Read the model definition and answer for the solid it produces. Units are mm, in the model's axes. Coordinates: 2 decimals unless noted, no trailing zeros. Write each loop counter-clockwise with the first axis right and the second up, starting at its lowest first coordinate (ties: lowest second). Pieces come first, ordered by that corner, then holes.
Item 1: Section C-C (z = -60) is taken. Give the vertices of the cut face in (x, y) (3 decimals), then the cut area to 3 significant figures.
Item 2: Section B-B (x = -34) is taken. Give the vertices of the cut face in (y, z) (3 decimals), then the cut area to 3 significant figures.
Item 3: Each of these flat-tipped pins is pushed along its axis until it touches: P1, Ø10, axis at x = 5.65, z = -53.34, coming from the +Y side (3 decimals); P2, Ø1, axis at y = 7.5, z = 74, coming from the -X side; P3, Ø5, axis at x = -40.5, y = 4, coming from the +Z side; P4, Ø5, axis at x = 38.5, y = 1.5, coming from the -Z side. Where does it stop, or does it pass through?
Item 4: Section A-A (z = 0) is taken. Give the vertices of the cut face in (x, y) (3 decimals).
Item 5: Section D-D (y = 7.5) is taken. State how many separate pieces and enclosed holes the cut face has, then the cut area to 3 significant figures.
Item 6: Straight lines are drawn through the part: probe 1 along Z at (x, y) = (57, 6); probe 2 along X at (y, z) = (1, 87); probe 3 along X at (y, z) = (7.75, 84.5). For each, find the intervals that lie inside material, in ascending order.
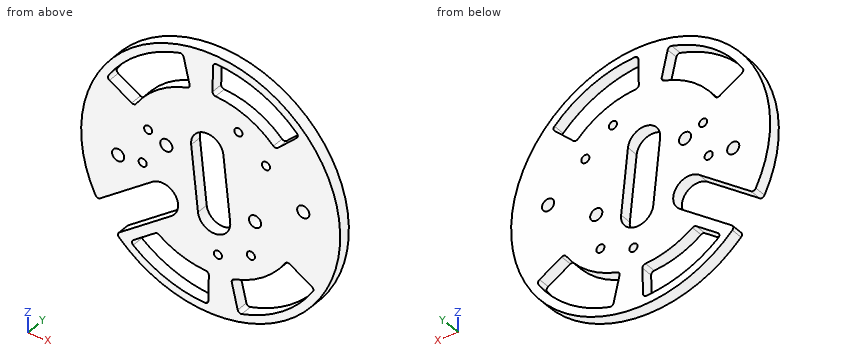
from build123d import *

# Parameters (mm, degrees)
SKETCH1_R           = 101.6
BOSS_EXTRUDE1_DEPTH = 9.525
SKETCH2_R           = 4.7625
SKETCH2_R_2         = 3.175
CUT_EXTRUDE1_DEPTH  = 22.86
SKETCH3_R           = 4.7625
CUT_EXTRUDE2_DEPTH  = 10.525
FILLET1_R           = 2.54
FILLET3_R           = 2.54


with BuildPart() as part:
    # Sketch1 → Boss-Extrude1 (new body)
    with BuildSketch(Plane(origin=(0, 0, 0), x_dir=(1, 0, 0), z_dir=(0, 1, 0))):
        Circle(SKETCH1_R)
    extrude(amount=BOSS_EXTRUDE1_DEPTH)

    # Sketch2 → Cut-Extrude1 (cut)
    with BuildSketch(Plane(origin=(0, 9.525, 0), x_dir=(1, 0, 0), z_dir=(0, 1, 0))):
        with BuildLine():
            Line((-9.955759688, 26.595729902), (-15.303128109, -23.922045692))
            ThreePointArc((-15.303128109, -23.922045692), (-4.010526316, -37.888331696), (9.955759688, -26.595729902))
            Line((9.955759688, -26.595729902), (15.303128109, 23.922045692))
            ThreePointArc((15.303128109, 23.922045692), (4.010526316, 37.888331696), (-9.955759688, 26.595729902))
        make_face()
        with Locations((34.817520913, 15.470948176)):
            Circle(SKETCH2_R)
        with Locations((-34.817520913, -15.470948176)):
            Circle(SKETCH2_R)
        with BuildLine():
            Line((-30.765292524, 38.093536125), (-87.237043764, 79.186441231))
            Line((-87.237043764, 79.186441231), (-104.485964967, 60.325))
            Line((-104.485964967, 60.325), (-45.710214871, 17.555539727))
            ThreePointArc((-45.710214871, 17.555539727), (-27.968755498, 20.352076753), (-30.765292524, 38.093536125))
        make_face()
        with Locations((5.646300897, 53.341856998)):
            Circle(SKETCH2_R_2)
        with Locations((31.560768513, 43.372252797)):
            Circle(SKETCH2_R_2)
        with Locations((-53.341856998, 5.646300897)):
            Circle(SKETCH2_R_2)
        with Locations((43.372252797, -31.560768513)):
            Circle(SKETCH2_R_2)
        with Locations((-49.018553694, -21.781088485)):
            Circle(SKETCH2_R_2)
        with Locations((21.781088485, -49.018553694)):
            Circle(SKETCH2_R_2)
    extrude(amount=-CUT_EXTRUDE1_DEPTH, mode=Mode.SUBTRACT)

    # Sketch3 → Cut-Extrude2 (cut, through all)
    with BuildSketch(Plane(origin=(0, 9.525, 0), x_dir=(1, 0, 0), z_dir=(0, 1, 0))):
        with BuildLine():
            ThreePointArc((15.979287148, 67.997682918), (41.099184753, 56.47901834), (59.78603337, 36.119976659))
            Line((59.78603337, 36.119976659), (81.526409141, 49.254513627))
            ThreePointArc((81.526409141, 49.254513627), (56.044342845, 77.016843191), (21.78993702, 92.72411307))
            Line((21.78993702, 92.72411307), (15.979287148, 67.997682918))
        make_face()
        with BuildLine():
            ThreePointArc((50.898077232, -47.837310063), (28.362672287, -63.832447241), (1.387800686, -69.83621202))
            Line((1.387800686, -69.83621202), (1.892455481, -95.231198209))
            ThreePointArc((1.892455481, -95.231198209), (38.6763713, -87.044246238), (69.406468953, -65.232695541))
            Line((69.406468953, -65.232695541), (50.898077232, -47.837310063))
        make_face()
        with BuildLine():
            ThreePointArc((-15.979287148, -67.997682918), (-41.099184753, -56.47901834), (-59.78603337, -36.119976659))
            Line((-59.78603337, -36.119976659), (-81.526409141, -49.254513627))
            ThreePointArc((-81.526409141, -49.254513627), (-56.044342845, -77.016843191), (-21.78993702, -92.72411307))
            Line((-21.78993702, -92.72411307), (-15.979287148, -67.997682918))
        make_face()
        with BuildLine():
            ThreePointArc((-42.080853774, 55.751450615), (-22.846796408, 66.00792675), (-1.387800686, 69.83621202))
            Line((-1.387800686, 69.83621202), (-1.892455481, 95.231198209))
            ThreePointArc((-1.892455481, 95.231198209), (-34.737758173, 88.689631058), (-63.288565419, 71.183705911))
            Line((-63.288565419, 71.183705911), (-42.080853774, 55.751450615))
        make_face()
        with Locations((-72.619302416, 7.686842105)):
            Circle(SKETCH3_R)
        with Locations((72.619302416, -7.686842105)):
            Circle(SKETCH3_R)
    extrude(amount=-CUT_EXTRUDE2_DEPTH, mode=Mode.SUBTRACT)

    # Fillet1
    fillet1_edges = [part.edges().sort_by_distance(p)[0] for p in [
        (-74.035185173, 4.7625, -69.579820037),
        (-88.980107519, 4.7625, -49.041823639),
    ]]
    fillet(fillet1_edges, radius=FILLET1_R)

    # Fillet3
    fillet3_edges = [part.edges().sort_by_distance(p)[0] for p in [
        (-15.979287148, 4.7625, 67.997682918),
        (-21.78993702, 4.7625, 92.72411307),
        (-81.526409141, 4.7625, 49.254513627),
        (-59.78603337, 4.7625, 36.119976659),
        (50.898077232, 4.7625, 47.837310063),
        (69.406468953, 4.7625, 65.232695541),
        (1.892455481, 4.7625, 95.231198209),
        (1.387800686, 4.7625, 69.83621202),
        (15.979287148, 4.7625, -67.997682918),
        (21.78993702, 4.7625, -92.72411307),
        (81.526409141, 4.7625, -49.254513627),
        (59.78603337, 4.7625, -36.119976659),
        (-42.080853774, 4.7625, -55.751450615),
        (-63.288565419, 4.7625, -71.183705911),
        (-1.892455481, 4.7625, -95.231198209),
        (-1.387800686, 4.7625, -69.83621202),
    ]]
    fillet(fillet3_edges, radius=FILLET3_R)


solid = part.part
Established:
1. outline: (-60.87, 0) - (-47.919, 0) - (-47.919, 9.525) - (-60.87, 9.525) - close; (-35.763, 0) - (35.763, 0) - (35.763, 9.525) - (-35.763, 9.525) - close; (73.977, 0) - (81.991, 0) - (81.991, 9.525) - (73.977, 9.525) - close
1. area: 881 mm2
2. outline: (0, -95.742) - (9.525, -95.742) - (9.525, -88.975) - (0, -88.975) - close; (0, -61.017) - (9.525, -61.017) - (9.525, -40.447) - (0, -40.447) - close; (0, -15.852) - (9.525, -15.852) - (9.525, 10.779) - (0, 10.779) - close; (0, 20.163) - (9.525, 20.163) - (9.525, 61.017) - (0, 61.017) - close; (0, 88.975) - (9.525, 88.975) - (9.525, 95.742) - (0, 95.742) - close
2. area: 968 mm2
3. P1: stops at y = 9.525
3. P2: stops at x = -70.14
3. P3: stops at z = 94.23
3. P4: stops at z = -95.01
4. outline: (-101.6, 0) - (-12.771, 0) - (-12.771, 9.525) - (-101.6, 9.525) - close; (12.771, 0) - (101.6, 0) - (101.6, 9.525) - (12.771, 9.525) - close
5. separate pieces: 1
5. enclosed holes: 15
5. area: 22,100 mm2
6. probe 1: z = -84.1 to -76.31, -40.37 to 53.57, 76.31 to 84.1
6. probe 2: x = -52.47 to -38.78, -20.44 to 1.73, 38.78 to 52.47
6. probe 3: x = -56.41 to -43.96, -19.86 to 1.68, 43.96 to 56.41
